Could you check a few things on this model? Use its own coordinates, in mm. Face numbers are marked on the shaded views. Give positions to 0.01 mm unless a question says otherwise; leave off trailing zeros. Write each loop counter-clockwise with the first axis right and the second up, starting at its lowest first coordinate (ties: lowest second). Pieces come first, ordered by that corner, then holes. Notation, with made-up numbers: (63, -23) - (76, -23) arc R32 ccw to (76, 15) - close; hole circle Ø8 at (-7, -11). An arc over 180 degrees is marked (long way). Answer in a Markdown table with one row per item.
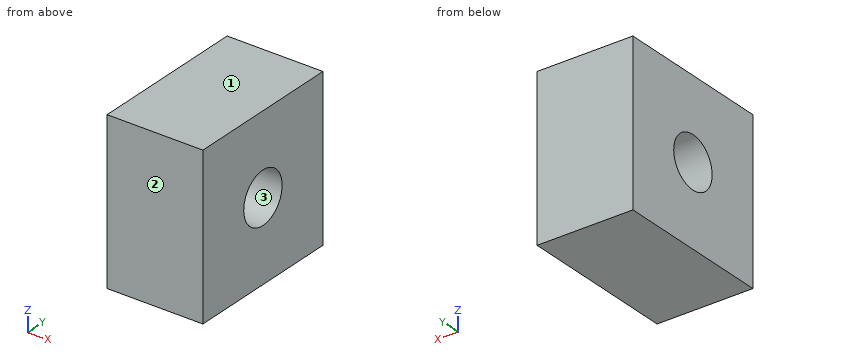
Autodesk Inventor part; units mm, degrees
ref_plane "Startebene" through (0, 0, 0) normal (0, 0, 1) x (1, 0, 0)
ref_plane "Endebene" through (0, 0, 50) normal (0, 0, 1) x (1, 0, 0)
ref_plane "YZ Plane" through (0, 0, 0) normal (1, 0, 0) x (0, 1, 0)
ref_plane "Startebene" through (0, 0, 0) normal (0, 0, 1) x (1, 0, 0)
ref_plane "Endebene" through (0, 0, 50) normal (0, 0, 1) x (1, 0, 0)
sketch "Skizze" plane through (0, 0, 0) normal (0, 0, 1) x (1, 0, 0)
  line L0 (15, -25) -> (-15, -25)
  line L1 (-15, -25) -> (-15, 25)
  line L2 (-15, 25) -> (15, 25)
  line L3 (15, 25) -> (15, -25)
  line L4 (-6, 0) -> (8, 0) construction
  line L5 (0, -30) -> (0, 40) construction
  line L6 (0, 54) -> (0, -44) construction
  line L7 (-9.2, 0) -> (13.2, 0) construction
  dimension "d0" = 50
  dimension "d1" = 30
  dimension "d4" = 15
  dimension "d5" = 25
extrude "Körper" add sketch "Skizze" along normal up to surface (50 mm away) from surface at 0
sketch "Sketch3" plane through (0, 0, 0) normal (0, 0, 1) x (1, 0, 0)
  line L0 (0, 0) -> (10, 0)
ref_plane "Work Plane3" through (0, 0, 0) normal (0, -1, 0) x (1, 0, 0)
sketch "Sketch4" plane through (0, 0, 0) normal (0, -1, 0) x (1, 0, 0)
  line L0 (-2, 0) -> (12, 0)
  line L1 (-2, 50) -> (12, 50)
  dimension "d9" = 50
sketch "Skizze5" plane through (15, -25, 50) normal (1, 0, 0) x (0, 0, -1)
  line L0 (0, 50) -> (0, 0)
  line L1 (50, 0) -> (0, 0)
  point P0 (50, 25)
  point P1 (25, 25)
  dimension "d10" = 25
  dimension "d11" = 25
hole "Bohrung1" at (15, 0, 25) direction (-1, 0, 0) diameter 16 end through all
equation "\"d0\" = G_W"
equation "\"d1\" = G_H"
equation "\"d4\" = 0.5 * d1"
equation "\"d5\" = 0.5 * d0"
equation "\"d2\" = G_L"
equation "\"G_W\" = 50"
equation "\"G_H\" = 30"
equation "\"G_L\" = d9"
equation "\"G_OFFSET_START\" = 0"
equation "\"G_OFFSET_END\" = 0"
properties part number "EN 10058 - 50 x 30 - 50" material "Stahl, weich"
1) Imagine slicing it at C-C (x = 3.25). List the corners of the cut face in (y, z) for me.
Check values:
| item | result |
|---|---|
| outline | (-25, 0) - (25, 0) - (25, 50) - (-25, 50) - close; hole circle Ø16 at (0, 25) |
2) We'd pull the mould along Y, two halves only. Please class the marked faces 1, 2 and 3: +Y half, -Y half, draft (parallel to the pull), parting line (faces both ways), or undercut.
Check values:
| item | result |
|---|---|
| face 1 | draft |
| face 2 | -Y half |
| face 3 | undercut |
3) Imagine slicing it at B-B (y = 0). List the corners of the cut face in (x, z) for me.
Check values:
| item | result |
|---|---|
| outline | (-15, 0) - (15, 0) - (15, 17) - (-15, 17) - close; (-15, 33) - (15, 33) - (15, 50) - (-15, 50) - close |
4) Imagine slicing it at A-A (z = 25). List the corners of the cut face in (x, y) for me, then the cut area to 3 significant figures.
Check values:
| item | result |
|---|---|
| outline | (-15, -25) - (15, -25) - (15, -8) - (-15, -8) - close; (-15, 8) - (15, 8) - (15, 25) - (-15, 25) - close |
| area | 1,020 mm2 |
5) If I drill on line 1 (Z direction, x = 5.5, y = 0); line 2 (Y direction, x = 0.5, z = 25); line 3 (Z direction, x = 11, y = 4), over which ranges is the centre line in solid material (lowest first)?
Check values:
| item | result |
|---|---|
| line 1 | z = 0 to 17, 33 to 50 |
| line 2 | y = -25 to -8, 8 to 25 |
| line 3 | z = 0 to 18.07, 31.93 to 50 |
6) Will this pin go through, and if not, where does the flat tip stop? P1, Ø21, axis at y = 0, z = 25, coming from the -X side.
Check values:
| item | result |
|---|---|
| P1 | stops at x = -15 |
